```python
from build123d import *

# Parameters (mm, degrees)
F1_W      = 21.5
F1_H      = 3.7829035334
F2_DEPTH  = 3
F0_W      = 21.5
F0_H      = 20
F3_DEPTH  = 1
F4_R      = 1
F5_DEPTH  = 21.5
F6_R      = 1
F7_DEPTH  = 4.75
F8_W      = 2.5
F8_H      = 2.5
F9_DEPTH  = 3
F11_DEPTH = 25


with BuildPart() as f2:
    # F1 (on face) → F2 (new body)
    with BuildSketch(Plane.XY):
        with Locations((0, 8.1085482333)):
            Rectangle(F1_W, F1_H)
    extrude(amount=-F2_DEPTH)

    # F0 (on Top) → F3 (join)
    with BuildSketch(Plane.XY):
        Rectangle(F0_W, F0_H)
    extrude(amount=F3_DEPTH)

    # F4 (on face) → F5 (cut)
    with BuildSketch(Plane(origin=(-10.75, 0, 0), x_dir=(0, -1, 0), z_dir=(-1, 0, 0))):
        with Locations((-8.1085482333, -1.5)):
            Circle(F4_R)
    extrude(amount=-F5_DEPTH, mode=Mode.SUBTRACT)

    # F6 (on Right) → F7 (join, symmetric)
    with BuildSketch(Plane.YZ):
        with BuildLine():
            ThreePointArc((-13.6414517667, 1), (-15.4092187197, 0.267766953), (-16.1414517667, -1.5))
            ThreePointArc((-16.1414517667, -1.5), (-14.3914517667, -3.25), (-12.6414517667, -1.5))
            ThreePointArc((-12.6414517667, -1.5), (-12.2021119385, -0.4393398282), (-11.1414517667, 0))
            Line((-11.1414517667, 0), (-10, 0))
            Line((-10, 0), (-10, 1))
            Line((-10, 1), (-13.6414517667, 1))
        make_face()
        with Locations((-14.3914517667, -1.5)):
            Circle(F6_R, mode=Mode.SUBTRACT)
        Polygon((10, 1), (-10, 1), (-10, 0), (6.2170964666, 0), (6.2170964666, -3), (10, -3), align=None)
        with Locations((8.1085482333, -1.5)):
            Circle(F6_R, mode=Mode.SUBTRACT)
    extrude(amount=F7_DEPTH, both=True)

    # F8 (on face) → F9 (join)
    with BuildSketch(Plane.XY.offset(1)):
        with Locations((-7.5, 11.25)):
            Rectangle(F8_W, F8_H)
        with Locations((7.5, 11.25)):
            Rectangle(F8_W, F8_H)
    extrude(amount=-F9_DEPTH)

    # F10 (on face) → F11 (cut)
    with BuildSketch(Plane(origin=(-8.75, 0, 0), x_dir=(0, -1, 0), z_dir=(-1, 0, 0))):
        with BuildLine():
            Line((-12.5, -2), (-10, -2))
            ThreePointArc((-10, -2), (-11.25, -1.2205063265), (-12.5, -2))
        make_face()
    extrude(amount=-F11_DEPTH, mode=Mode.SUBTRACT)


solid = f2.part
```
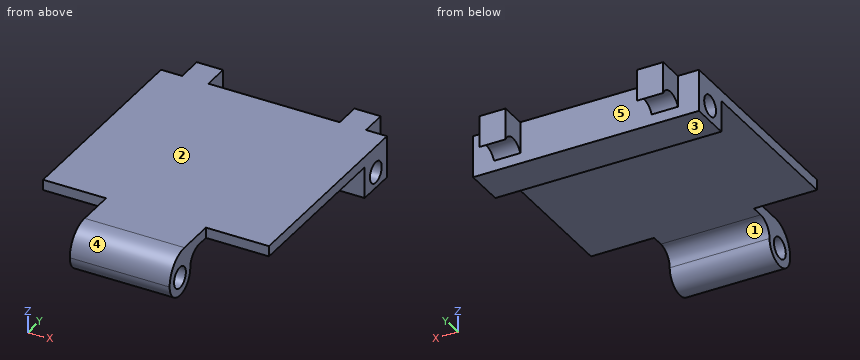
Check sheet for the modelled part. Datum: model origin and axes. Units: mm. Face numbers are marked on the shaded views. A direction names the side the tool comes from. Round coordinates to 2 decimals unless told otherwise and drop trailing zeros. Write each loop counter-clockwise with the first axis right and the second up, starting at its lowest first coordinate (ties: lowest second). Pieces come first, ordered by that corner, then holes. Notation, with made-up numbers: M 32,63 L 77,63 A28 cw 77,95 Z; hole C 8.5,23 d1. An arc over 180 degrees is marked long. Write item = value, one per line. Start each with the question number.
1. Section check D-D, the plane x = -9.5. Record the cut outline in (y, z), then the cut area to 3 significant figures.
2. Section check B-B, the plane x = -1. Record the cut outline in (y, z).
3. Scan lines: line 1 (Y direction, x = -3.5, z = -1.45); line 2 (Y direction, x = 1, z = -2.3); line 3 (Y direction, x = -8.5, z = -2.85). Record each from-to range of solid material in increasing order. Write a range as [from, to].
4. Gauge pin test, flat ends, axial feed: pin 1 (2.5 mm diameter, centred on x = 0.5, z = -2, fed in from -Y); pin 2 (2 mm diameter, centred on x = -5, z = -1, fed in from +Y); pin 3 (10 mm diameter, centred on x = 7, y = 7, fed in from -Z); pin 4 (1.1 mm diameter, centred on x = -7.5, z = 0.5, fed in from -Y). Record the tip position at first contact, or that the pin passes through.
5. Section check A-A, the plane x = 7.25. Record the cut outline in (y, z).
6. Section check C-C, the plane z = 0.4. Record the cut outline in (x, y).
7. Tool access check on the marked faces 1, 2 and 3. Record the directions out of +Z, -Z, +X, -X, +Y, -Y that give a thin tool (end or side, any length) a straight path to the whole face; none if there is none.
8. Release check for a two-part mould opening along X. For the marked faces 4 and 5 record: pulls with the +X half, pulls with the -X half, needs draft (parallel to the pull), parting line crosses it, or undercut.
Results found:
q1.outline = M -10,0 L 6.22,0 L 6.22,-3 L 10,-3 L 10,1 L -10,1 Z; hole C 8.11,-1.5 d2
q1.area = 28.2 mm^2
q2.outline = M -16.14,-1.5 A1.75 ccw -12.64,-1.5 A1.5 cw -11.14,0 L 6.22,0 L 6.22,-3 L 10,-3 L 10,1 L -13.64,1 A2.5 ccw Z; hole C -14.39,-1.5 d2; hole C 8.11,-1.5 d2
q3.line_1 = [-16.14, -15.39], [-13.39, -12.64], [6.22, 7.11], [9.11, 10]
q3.line_2 = [-15.95, -14.99], [-13.79, -12.84], [6.22, 7.51], [8.71, 10]
q3.line_3 = [6.22, 10]
q4.pin_1 = -16.14
q4.pin_2 = 10
q4.pin_3 = -3
q4.pin_4 = -10
q5.outline = M -10,0 L 6.22,0 L 6.22,-3 L 10,-3 L 10,-2 A1.39 cw 12.5,-2 L 12.5,1 L -10,1 Z; hole C 8.11,-1.5 d2
q6.outline = M -10.75,-10 L -4.75,-10 L -4.75,-15.27 L 4.75,-15.27 L 4.75,-10 L 10.75,-10 L 10.75,10 L 8.75,10 L 8.75,12.5 L 6.25,12.5 L 6.25,10 L -6.25,10 L -6.25,12.5 L -8.75,12.5 L -8.75,10 L -10.75,10 Z
q7.face_1 = -Z, +X, -X
q7.face_2 = +Z, +X, -X, +Y, -Y
q7.face_3 = -Z, +X, -X, +Y
q8.face_4 = needs draft
q8.face_5 = undercut
